Read the model definition and answer for the solid it produces. Units are mm, in the model's axes. Give positions to 0.01 mm unless a question says otherwise; leave off trailing zeros. Order: outer loops, then holes, each group sorted by start corner. A loop starts at its lowest first (then second) coordinate and runs counter-clockwise, first axis right, second up. Notation, with made-up numbers: (53, -38) -> (58, -38) arc R32 ccw to (58, -8) -> close; hole circle Ø1 at (-8, 59). An arc over 180 degrees is marked (long way). One line per item, written item: value. Start each with the question number.
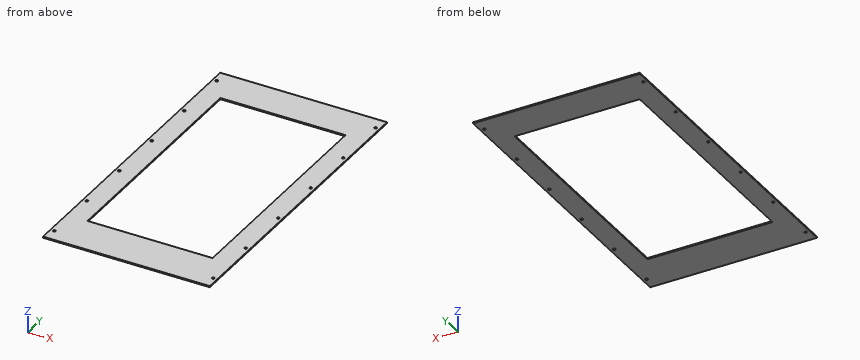
Autodesk Inventor part; units mm, degrees
ref_plane "YZ Plane" through (0, 0, 0) normal (1, 0, 0) x (0, 1, 0)
ref_plane "XZ Plane" through (0, 0, 0) normal (0, 1, 0) x (-1, 0, 0)
ref_plane "XY Plane" through (0, 0, 0) normal (0, 0, 1) x (1, 0, 0)
sketch "Sketch1" plane through (0, 0, 0) normal (0, 0, 1) x (1, 0, 0)
  line L0 (-203.2, 381) -> (203.2, 381)
  line L1 (203.2, 381) -> (203.2, -381)
  line L2 (203.2, -381) -> (-203.2, -381)
  line L3 (-203.2, -381) -> (-203.2, 381)
  point P0 (0, 0)
  point P1 (203.2, 0)
  point P2 (0, 381)
  dimension "d0" = 406.4
  dimension "d1" = 762
extrude "Extrusion1" add sketch "Sketch1" along normal blind 3
sketch "Sketch2" plane through (0, 0, 3) normal (0, 0, 1) x (1, 0, 0)
  line L0 (203.2, 381) -> (203.2, -381)
  line L1 (-203.2, -381) -> (-203.2, 381)
  line L2 (203.2, -381) -> (-203.2, -381)
  line L3 (-152.4, 292.1) -> (152.4, 292.1)
  line L4 (152.4, 292.1) -> (152.4, -279.4)
  line L5 (152.4, -279.4) -> (-152.4, -279.4)
  line L6 (-152.4, -279.4) -> (-152.4, 292.1)
  point P0 (0, 0)
  dimension "d4" = 101.6
  dimension "d5" = 50.8
  dimension "d6" = 571.5
  dimension "d7" = 50.8
extrude "Extrusion2" cut sketch "Sketch2" against normal blind 3
sketch "Sketch3" plane through (0, 0, 3) normal (0, 0, 1) x (1, 0, 0)
  line L0 (-203.2, 381) -> (203.2, 381)
  line L1 (-203.2, -381) -> (-203.2, 381)
  line L2 (203.2, -381) -> (-203.2, -381)
  line L3 (0, 473.1075) -> (0, -607.181)
  point P0 (0, 0)
  point P1 (-193.675, 349.25)
  point P2 (-193.675, 209.55)
  point P3 (-193.675, 69.85)
  point P4 (-193.675, -69.85)
  point P5 (-193.675, -209.55)
  point P6 (-193.675, -349.25)
  point P7 (193.675, 349.25)
  point P8 (193.675, 209.55)
  point P9 (193.675, 69.85)
  point P10 (193.675, -69.85)
  point P11 (193.675, -209.55)
  point P12 (193.675, -349.25)
  dimension "d10" = 31.75
  dimension "d11" = 9.525
  dimension "d25" = 139.7
  dimension "d26" = 139.7
  dimension "d27" = 139.7
  dimension "d28" = 139.7
  dimension "d29" = 139.7
hole "Hole2" at (-193.675, 349.25, 3) at (-193.675, 209.55, 3) at (-193.675, 69.85, 3) at (-193.675, -69.85, 3) at (-193.675, -209.55, 3) at (-193.675, -349.25, 3) at (193.675, 349.25, 3) at (193.675, 209.55, 3) at (193.675, 69.85, 3) at (193.675, -69.85, 3) at (193.675, -209.55, 3) at (193.675, -349.25, 3) direction (0, 0, -1) diameter 6.35 end through all
properties part number "front cover"
Item 1: Find section B-B on y = -149.5. Write down the section's boundary in (x, z).
Item 2: Find section A-A on x = -2. Write down the section's boundary in (y, z).
Item 3: Find section C-C on z = 1.8. Count the separate pieces of the cut face and the enclosed holes in it, then the cut area to 3 significant figures.
Item 4: Find the intervals of material crossed by line 1 (X direction, y = -349.25, z = 1.05); line 2 (X direction, y = -209.55, z = 2.45); line 3 (X direction, y = -12, z = 0.7), in increasing order. Write a range as from..to.
Checks:
1. outline: (-203.2, 0) -> (-152.4, 0) -> (-152.4, 3) -> (-203.2, 3) -> close; (152.4, 0) -> (203.2, 0) -> (203.2, 3) -> (152.4, 3) -> close
2. outline: (-381, 0) -> (-279.4, 0) -> (-279.4, 3) -> (-381, 3) -> close; (292.1, 0) -> (381, 0) -> (381, 3) -> (292.1, 3) -> close
3. separate pieces: 1
3. enclosed holes: 13
3. area: 135,000 mm2
4. line 1: -203.2..-196.85, -190.5..190.5, 196.85..203.2
4. line 2: -203.2..-196.85, -190.5..-152.4, 152.4..190.5, 196.85..203.2
4. line 3: -203.2..-152.4, 152.4..203.2
